Input: part model. Units: mm. Frame: model coordinates. Face numbers are marked on the shaded views. Round coordinates to 2 decimals unless told otherwise and drop trailing zeros. Loops run counter-clockwise (first coordinate to the right, second up) from the corner with the lowest first, then second, coordinate; pieces in that order, holes last. Notation, with made-up numbers: (69.25, -25.75) -> (102.25, -25.75) arc R31 ccw to (102.25, 6.25) -> close; hole circle Ø3 at (46, 52.25). An arc over 180 degrees is marked (long way). Answer in a Markdown table with one row per item. Add a question column.
Q1. Section B-B, the plane x = 0. Output: boundary loops of the cut face in (y, z), and give its area (3 significant figures).
Q2. Ray query, L1, parallel to X at y = 7, z = 0; L2, parallel to Y at x = 2, z = 1.5. Return the intervals inside material, ascending. Write a range as from..to.
Q3. Mould query, pull axis X, two halves, no side actions, for the marked faces 1, 2 and 3. Classes: pulls with the +X half, pulls with the -X half, needs draft (parallel to the pull), parting line crosses it, or undercut.
Q4. Pin query (flat end, axial travel): pin 1 (4 mm diameter, centred on x = -2.5, y = 7.5, fed in from -Z); pin 2 (6 mm diameter, centred on y = 7, z = -3, fed in from +X); pin 3 (2 mm diameter, centred on x = -2.5, y = 2, fed in from -Z); pin 4 (1.5 mm diameter, centred on x = 11, y = 9, fed in from -Z). Return the tip coordinate at first contact, or that it passes through.
Q5. Section A-A, the plane z = 0. Output: boundary loops of the cut face in (x, y).
Q6. Section C-C, the plane y = 4.5. Output: boundary loops of the cut face in (x, z), and give its area (3 significant figures).
```python
from build123d import *

# Parameters (mm, degrees)
SKETCH1_R           = 18
BOSS_EXTRUDE1_DEPTH = 10
SKETCH2_R           = 1.55
SKETCH4_R           = 3
CUT_EXTRUDE1_DEPTH  = 8


with BuildPart() as part:
    # Sketch1 → Boss-Extrude1 (new body)
    with BuildSketch(Plane(origin=(0, 0, 0), x_dir=(1, 0, 0), z_dir=(0, 1, 0))):
        Circle(SKETCH1_R)
    extrude(amount=BOSS_EXTRUDE1_DEPTH)

    # Sketch2 → Cut-Revolve1 (revolve, cut)
    with BuildSketch(Plane.XY):
        with Locations((18, 3.5)):
            Circle(SKETCH2_R)
    revolve(axis=Axis((0, 0, 0), (0, 1, 0)), mode=Mode.SUBTRACT)

    # Sketch4 → Cut-Extrude1 (cut)
    with BuildSketch(Plane(origin=(0, 10, 0), x_dir=(1, 0, 0), z_dir=(0, 1, 0))):
        Circle(SKETCH4_R)
    extrude(amount=-CUT_EXTRUDE1_DEPTH, mode=Mode.SUBTRACT)


solid = part.part
```
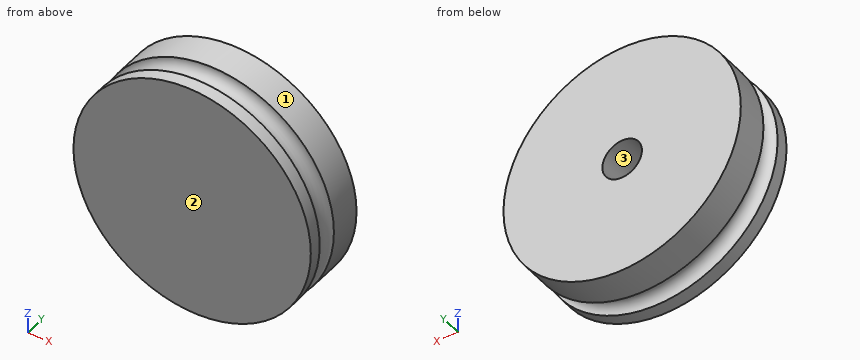
Answer block:
| question | item | result |
|---|---|---|
| 1 | outline | (0, -18) -> (1.95, -18) arc R1.55 cw to (5.05, -18) -> (10, -18) -> (10, -3) -> (2, -3) -> (2, 3) -> (10, 3) -> (10, 18) -> (5.05, 18) arc R1.55 cw to (1.95, 18) -> (0, 18) -> close |
| 1 | area | 304 mm^2 |
| 2 | L1 | -18..-3, 3..18 |
| 2 | L2 | 0..2 |
| 3 | face 1 | parting line crosses it |
| 3 | face 2 | needs draft |
| 3 | face 3 | undercut |
| 4 | pin 1 | z = -17.99 |
| 4 | pin 2 | x = 18 |
| 4 | pin 3 | z = -17.94 |
| 4 | pin 4 | z = -14.8 |
| 5 | outline | (-18, 0) -> (18, 0) -> (18, 1.95) arc R1.55 cw to (18, 5.05) -> (18, 10) -> (3, 10) -> (3, 2) -> (-3, 2) -> (-3, 10) -> (-18, 10) -> (-18, 5.05) arc R1.55 cw to (-18, 1.95) -> close |
| 6 | outline | circle Ø33.63 at (0, 0); hole circle Ø6 at (0, 0) |
| 6 | area | 860 mm^2 |
